Autodesk Inventor part; units mm, degrees
ref_plane "YZ Plane" through (0, 0, 0) normal (1, 0, 0) x (0, 1, 0)
ref_plane "XZ Plane" through (0, 0, 0) normal (0, 1, 0) x (-1, 0, 0)
ref_plane "XY Plane" through (0, 0, 0) normal (0, 0, 1) x (1, 0, 0)
sketch "Sketch1" plane through (0, 0, 0) normal (0, 0, 1) x (1, 0, 0)
  arc A0 (6.0128, 43.747) -> (6.9228, 42.8627) centre (5.7994, 42.6169) ccw
  arc A1 (6.2634, 45.0735) -> (8.2994, 42.6027) centre (5.7994, 42.6169) ccw
  arc A2 (19.5106, 33.7857) -> (21.381, 31.3359) centre (18.8812, 31.3663) ccw
  line L0 (6.2634, 45.0735) -> (9.5295, 44.4566)
  line L1 (9.5295, 44.4566) -> (21.4782, 39.3353)
  line L2 (21.4782, 39.3353) -> (21.381, 31.3359)
  line L3 (6.0128, 43.747) -> (9.3605, 43.1146)
  line L4 (9.3605, 43.1146) -> (20.2673, 38.4399)
  line L5 (20.2673, 38.4399) -> (20.1811, 31.3505)
  line L6 (6.9228, 42.8627) -> (8.2994, 42.6027)
  line L7 (19.5106, 33.7857) -> (19.4952, 32.5121)
  arc A3 (19.4952, 32.5121) -> (20.1811, 31.3505) centre (18.8812, 31.3663) ccw
  line L8 (5.7994, 42.6169) -> (18.8812, 31.3663) construction
  arc A4 (6.9392, 42.2416) -> (4.6204, 42.3936) centre (5.7994, 42.6169) ccw
  point P0 (0, 0)
  dimension "d0" = 5
  dimension "d1" = 5
  dimension "d2" = 1.3
  dimension "d5" = 1.35
  dimension "d8" = 8
  dimension "d9" = 0.7
  dimension "d10" = 0.7
  dimension "d12" = 1.2
  dimension "d18" = 2.3
  dimension "d19" = 30
  dimension "d20" = 13
  dimension "d21" = 50
extrude "Extrusion1" add sketch "Sketch1" along normal mid plane 10 contours A0 L6 A1 L0 L1 L2 A2 L7 A3 L5 L4 L3
fillet "Fillet1" radius 2 2 edges at (20.2673, 38.4399, 0) (9.3605, 43.1146, 0)
fillet "Fillet1" radius 3 2 edges at (9.5295, 44.4566, 0) (21.4782, 39.3353, 0)
properties part number "Linkage for half overlay hinge" material "Steel"
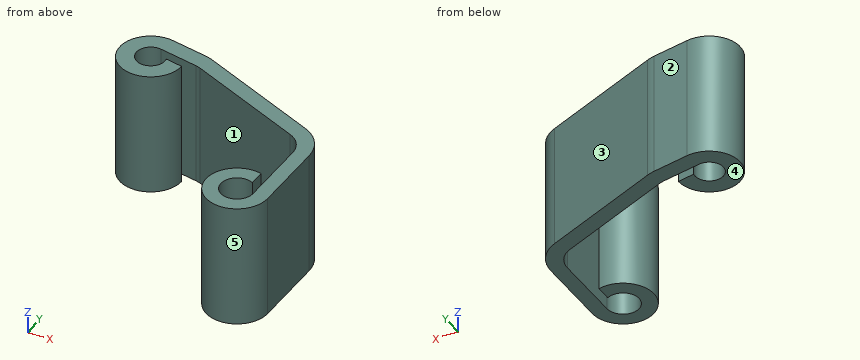
Build history of the part. All positions in model axes, mm. Face numbers are marked on the shaded views. A direction names the side the tool comes from. Coordinates: 2 decimals unless noted, no trailing zeros. Write each loop counter-clockwise with the first axis right and the second up, starting at its lowest first coordinate (ties: lowest second). Pieces come first, ordered by that corner, then holes.
1. Band-saw the part on A-A, the plane x = 18.5. Give the cut face in (y, z), and give its area (3 significant figures).
Answer block:
outline: (28.9, -5) - (30.12, -5) - (30.12, 5) - (28.9, 5) - close; (32.61, -5) - (33.84, -5) - (33.84, 5) - (32.61, 5) - close; (39.2, -5) - (40.61, -5) - (40.61, 5) - (39.2, 5) - close
area: 38.7 mm2
2. 3-axis set-ups, long thin cutter, end or side, ignore diameter. For the marked faces 1 and 2: which of +Z, -Z, +X, -X, +Y, -Y reach the whole face in a straight line?
Answer block:
face 1: +Z, -Z
face 2: +Z, -Z, +X, +Y
3. Band-saw the part on C-C, the plane y = 40.5. Give the cut face in (x, z), and give its area (3 significant figures).
Answer block:
outline: (4.47, -5) - (7.13, -5) - (7.13, 5) - (4.47, 5) - close; (15.46, -5) - (18.76, -5) - (18.76, 5) - (15.46, 5) - close
area: 59.6 mm2
4. Band-saw the part on D-D, the plane x = 5. Give the cut face in (y, z).
Answer block:
outline: (40.25, -5) - (41.79, -5) - (41.79, 5) - (40.25, 5) - close; (43.44, -5) - (44.99, -5) - (44.99, 5) - (43.44, 5) - close
5. Pull direction Y, two halves, no side cores. Call the marked faces 3, 4 and 5: released by +Y, released by -Y, zero draft, split by the parting line, or undercut.
Answer block:
face 3: released by +Y
face 4: zero draft
face 5: undercut
6. Drill centre lines: probe 1 along Y at (x, z) = (18.25, -1); probe 2 along Y at (x, z) = (17.25, 2); probe 3 along Y at (x, z) = (8, 1). Where is each one in solid material? Low to high.
Answer block:
probe 1: y = 28.95 to 30.23, 32.5 to 33.79, 39.3 to 40.72
probe 2: y = 29.47 to 33.26, 39.73 to 41.15
probe 3: y = 41.43 to 42.66, 43.37 to 44.75
7. Drop flat-ended pins along their axis: pin 1 (2 mm diameter, centred on y = 39, z = -2.5, fed in from -X); pin 2 (1 mm diameter, centred on x = 18.5, z = 3.5, fed in from +Y); pin 3 (6 mm diameter, centred on y = 38.5, z = 2.5, fed in from -X). Give the stop position or say it passes through.
Answer block:
pin 1: stops at x = 16.63
pin 2: stops at y = 40.83
pin 3: stops at x = 3.56
8. Band-saw the part on B-B, the plane z = -3.25. Give the cut face in (x, y), and give its area (3 significant figures).
Answer block:
outline: (6.01, 43.75) - (9.15, 43.16) arc R2 cw to (9.56, 43.03) - (19.04, 38.97) arc R2 cw to (20.25, 37.1) - (20.18, 31.35) arc R1.3 cw (long way) to (19.5, 32.51) - (19.51, 33.79) arc R2.5 ccw (long way) to (21.38, 31.34) - (21.45, 37.33) arc R3 ccw to (19.64, 40.12) - (9.83, 44.33) arc R3 ccw to (9.21, 44.52) - (6.26, 45.07) arc R2.5 ccw (long way) to (8.3, 42.6) - (6.92, 42.86) arc R1.15 cw (long way) to start
area: 53.1 mm2
